```python
from build123d import *

# Parameters (mm, degrees)
SKETCH1_R           = 2.286
BOSS_EXTRUDE1_DEPTH = 3.175
SKETCH2_R           = 2.20991013
CUT_EXTRUDE1_DEPTH  = 58.875643193


with BuildPart() as part:
    # Sketch1 → Boss-Extrude1 (new body)
    with BuildSketch(Plane(origin=(0, 0, 0), x_dir=(0, 0, -1), z_dir=(1, 0, 0))):
        with BuildLine():
            Line((1.386091097, 11.894364388), (52.186091097, -0.805635612))
            ThreePointArc((52.186091097, -0.805635612), (56.472180686, -7.048277352), (50.8, -12.065))
            Line((50.8, -12.065), (0, -12.065))
            Line((0, -12.065), (-41.91, -12.065))
            ThreePointArc((-41.91, -12.065), (-43.706051224, -11.321051224), (-44.45, -9.525))
            Line((-44.45, -9.525), (-44.45, 9.525))
            ThreePointArc((-44.45, 9.525), (-43.706051224, 11.321051224), (-41.91, 12.065))
            Line((-41.91, 12.065), (0, 12.065))
            ThreePointArc((0, 12.065), (0.698277352, 12.022180686), (1.386091097, 11.894364388))
        make_face()
        with Locations((0, 6.35)):
            Circle(SKETCH1_R, mode=Mode.SUBTRACT)
        with Locations((0, -6.35)):
            Circle(SKETCH1_R, mode=Mode.SUBTRACT)
        with Locations((50.8, -6.35)):
            Circle(SKETCH1_R, mode=Mode.SUBTRACT)
    extrude(amount=BOSS_EXTRUDE1_DEPTH)

    # Sketch2 → Cut-Extrude1 (cut, through all)
    with BuildSketch(Plane(origin=(3.175, 0, 0), x_dir=(0, 0, -1), z_dir=(1, 0, 0))):
        with Locations((-37.310316922, 6.68008987)):
            Circle(SKETCH2_R)
        with Locations((-37.310316922, -6.68008987)):
            Circle(SKETCH2_R)
    extrude(amount=-CUT_EXTRUDE1_DEPTH, mode=Mode.SUBTRACT)


solid = part.part
```
Geometry check sheet. Reference: the model listing, model coordinates, mm. Coordinates: 2 decimals unless noted, no trailing zeros. Loops run counter-clockwise (first coordinate to the right, second up) from the corner with the lowest first, then second, coordinate; pieces in that order, holes last. Notation, with made-up numbers: (-31, -23) - (-7, -23) arc R27 cw to (-7, 0) - close; hole circle Ø2 at (-4, 11). An arc over 180 degrees is marked (long way). One line per item, written item: value. Start each with the question number.
(1) Cross-section at C-C on y = 0.75. Enter the section's corners in (x, z) (3 decimals), plus the area to 3 significant figures.
(2) Mould release check, pull along Z, two halves, no side actions. Record for faces 1 (the flat face through (0, -3, 4)), 2 (the cylindrical face through (1.61, -6.583, 39.518)), 3 (the flat face through (1.565, 5.633, -26.43)): released by +Z, released by -Z, zero draft, split by the parting line, or undercut.
(3) Cross-section at A-A on x = 0.7. Enter the section's corners in (y, z) (3 decimals), plus the area to 3 significant figures.
(4) Cross-section at B-B on z = -16. Enter the section's corners in (x, y) (3 decimals).
(5) Material ranges on line 1 (Y direction, x = 2.1, z = 0) (3 decimals); line 2 (Z direction, x = 2, y = -8); line 3 (Z direction, x = 1.25, y = -11), recorded low to high. Write a range as [from, to].
Results below:
1. outline: (0, -45.964) - (3.175, -45.964) - (3.175, 44.45) - (0, 44.45) - close
1. area: 287 mm2
2. face 1: zero draft
2. face 2: undercut
2. face 3: released by -Z
3. outline: (-12.065, -50.8) arc R5.715 ccw to (-0.806, -52.186) - (11.894, -1.386) arc R5.715 ccw to (12.065, 0) - (12.065, 41.91) arc R2.54 ccw to (9.525, 44.45) - (-9.525, 44.45) arc R2.54 ccw to (-12.065, 41.91) - close; hole circle Ø4.42 at (-6.68, 37.31); hole circle Ø4.572 at (-6.35, -50.8); hole circle Ø4.572 at (-6.35, 0); hole circle Ø4.572 at (6.35, 0); hole circle Ø4.42 at (6.68, 37.31)
3. area: 1,950 mm2
4. outline: (0, -12.065) - (3.175, -12.065) - (3.175, 8.241) - (0, 8.241) - close
5. line 1: y = [-12.065, -8.636], [-4.064, 4.064], [8.636, 12.065]
5. line 2: z = [-56.27, -52.38], [-49.22, -1.58], [1.58, 35.54], [39.08, 44.45]
5. line 3: z = [-54.12, 43.98]
